Part model, mm, in its own coordinate system. A direction names the side the tool comes from. Round coordinates to 2 decimals unless told otherwise and drop trailing zeros. Use a Markdown table: item, result. Add a question column.
1) Drop flat-ended pins along their axis: P1, Ø0.5, axis at y = -15.5, z = -1, coming from the -X side; P2, Ø4, axis at y = 23.5, z = -18, coming from the -X side; P3, Ø0.8, axis at x = 8, z = -1, coming from the -Y side. Give the stop position or say it passes through.
2) Wall check: probe 1 along Z at (x, y) = (30.5, 0.5) (3 decimals); probe 2 along Y at (x, z) = (-52.5, -5.5); probe 3 along X at (y, z) = (6, -20). Give the ranges that are in metal, low to high.
3) Which spindle directions (+Z, -Z, +X, -X, +Y, -Y) get a long thin tool onto all of the face, cutting with end or side? Do faces 1 (the face through (-5.4, 32.5, 0)), 2 (the face through (-1, 0, -1.524)). Say none if no direction does.
```python
from build123d import *

# Parameters (mm, degrees)
F0_W          = 128.016
F0_H          = 67.564
F1_DEPTH      = 28.575
F1_TAPER      = -5
F2_W          = 2.4999885603
F2_H          = 28.575
F3_DEPTH      = 66.5089886603
F3_DEPTH_BACK = 66.5089886603
F4_W          = 124.968
F4_H          = 66.04
F5_DEPTH      = 1.524


with BuildPart() as f1:
    # F0 (on Top) → F1 (new body)
    with BuildSketch(Plane.XY):
        Rectangle(F0_W, F0_H)
    extrude(amount=-F1_DEPTH, taper=F1_TAPER)

    # F2 (on Right) → F3 (cut, two sides)
    with BuildSketch(Plane.YZ) as f3_sk:
        with Locations((-35.0319942801, -14.2875)):
            Rectangle(F2_W, F2_H)
    extrude(amount=-F3_DEPTH, mode=Mode.SUBTRACT)
    extrude(f3_sk.sketch, amount=F3_DEPTH_BACK, mode=Mode.SUBTRACT)

    # F4 (on face) → F5 (cut)
    with BuildSketch(Plane.XY):
        with Locations((0, -0.762)):
            Rectangle(F4_W, F4_H)
    extrude(amount=-F5_DEPTH, mode=Mode.SUBTRACT)


solid = f1.part
```
Entries:
| question | item | result |
|---|---|---|
| 1 | P1 | stops at x = -64.12 |
| 1 | P2 | stops at x = -65.76 |
| 1 | P3 | stops at y = 32.26 |
| 2 | probe 1 | z = -28.575 to -1.524 |
| 2 | probe 2 | y = -33.78 to 34.26 |
| 2 | probe 3 | x = -65.76 to 65.76 |
| 3 | face 1 | +Z, +X, -X, +Y, -Y |
| 3 | face 2 | +Z, -Y |
